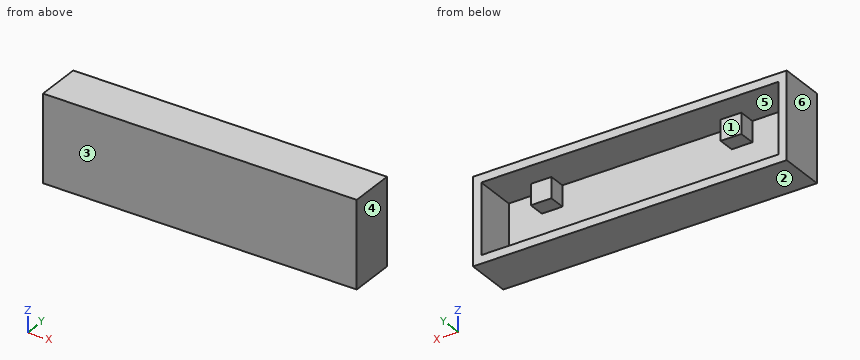
from build123d import *

# Parameters (mm, degrees)
SKETCH1_W           = 76
SKETCH1_H           = 21
SKETCH1_W_2         = 72
SKETCH1_H_2         = 17
BOSS_EXTRUDE1_DEPTH = 10
SKETCH2_W           = 76
SKETCH2_H           = 21
BOSS_EXTRUDE2_DEPTH = 1
SKETCH3_W           = 3.936198622
SKETCH3_H           = 4.059160528
SKETCH3_W_2         = 4.339911302
BOSS_EXTRUDE3_DEPTH = 4
SKETCH4_W           = 5
SKETCH4_H           = 5
BOSS_EXTRUDE4_DEPTH = 4


with BuildPart() as part:
    # Sketch1 → Boss-Extrude1 (new body)
    with BuildSketch(Plane(origin=(0, 0, 0), x_dir=(1, 0, 0), z_dir=(0, 1, 0))):
        with Locations((36, 8.5)):
            Rectangle(SKETCH1_W, SKETCH1_H)
        with Locations((36, 8.5)):
            Rectangle(SKETCH1_W_2, SKETCH1_H_2, mode=Mode.SUBTRACT)
    extrude(amount=BOSS_EXTRUDE1_DEPTH)

    # Sketch2 → Boss-Extrude2 (add)
    with BuildSketch(Plane.XZ):
        with Locations((36, -8.5)):
            Rectangle(SKETCH2_W, SKETCH2_H)
    extrude(amount=BOSS_EXTRUDE2_DEPTH)

    # Sketch3 → Boss-Extrude3 (add)
    with BuildSketch(Plane(origin=(0, 0, 0), x_dir=(1, 0, 0), z_dir=(0, 1, 0))):
        with Locations((18.943139302, 14.970419736)):
            Rectangle(SKETCH3_W, SKETCH3_H)
        with Locations((52.653148019, 14.970419736)):
            Rectangle(SKETCH3_W_2, SKETCH3_H)
    extrude(amount=BOSS_EXTRUDE3_DEPTH)

    # Sketch4 → Boss-Extrude4 (add)
    with BuildSketch(Plane(origin=(0, 0, 0), x_dir=(1, 0, 0), z_dir=(0, 1, 0))):
        with Locations((15.5, 2.5)):
            Rectangle(SKETCH4_W, SKETCH4_H)
        with Locations((61.5, 2.5)):
            Rectangle(SKETCH4_W, SKETCH4_H)
    extrude(amount=BOSS_EXTRUDE4_DEPTH)


solid = part.part
CAD build for the part. Positions are in the model's coordinates, mm. Face numbers are marked on the shaded views. A direction names the side the tool comes from. Give positions to 0.01 mm unless a question says otherwise; leave off trailing zeros. Write each loop counter-clockwise with the first axis right and the second up, starting at its lowest first coordinate (ties: lowest second). Pieces come first, ordered by that corner, then holes. Notation, with made-up numbers: (1.25, 59.5) -> (51.25, 59.5) arc R23 cw to (51.25, 89.5) -> close; hole circle Ø4 at (32, -23.5). An arc over 180 degrees is marked (long way). Return JSON: item names as keys, results as strings.
Item 1: Drop flat-ended pins along their axis: pin 1 (4.5 mm diameter, centred on x = 53.5, z = -15, fed in from +Y); pin 2 (5.5 mm diameter, centred on x = 15, z = -3.5, fed in from +Y); pin 3 (6 mm diameter, centred on x = 38, z = -3.5, fed in from +Y). Give the stop position or say it passes through.
Answer below:
{"pin 1": "stops at y = 10", "pin 2": "stops at y = 4", "pin 3": "stops at y = 0"}
Item 2: Drill centre lines: probe 1 along X at (y, z) = (1.5, -16.25); probe 2 along X at (y, z) = (3.75, -2.75); probe 3 along Z at (x, y) = (51, 3.5). Where is each one in solid material? Low to high.
Answer below:
{"probe 1": "x = -2 to 0, 16.98 to 20.91, 50.48 to 54.82, 72 to 74", "probe 2": "x = -2 to 0, 13 to 18, 59 to 64, 72 to 74", "probe 3": "z = -19 to -12.94, 0 to 2"}
Item 3: Band-saw the part on D-D (y = 3). List the corners of the cut face in (x, z).
Answer below:
{"outline": "(-2, -19) -> (74, -19) -> (74, 2) -> (-2, 2) -> close; hole (0, -17) -> (16.98, -17) -> (16.98, -12.94) -> (20.91, -12.94) -> (20.91, -17) -> (50.48, -17) -> (50.48, -12.94) -> (54.82, -12.94) -> (54.82, -17) -> (72, -17) -> (72, 0) -> (64, 0) -> (64, -5) -> (59, -5) -> (59, 0) -> (18, 0) -> (18, -5) -> (13, -5) -> (13, 0) -> (0, 0) -> close"}
Item 4: Band-saw the part on C-C (z = -10.25). List the corners of the cut face in (x, y).
Answer below:
{"outline": "(-2, -1) -> (74, -1) -> (74, 10) -> (72, 10) -> (72, 0) -> (0, 0) -> (0, 10) -> (-2, 10) -> close"}
Item 5: Two-plate mould, pull along X, no slides. Class the marked faces 3, 4, 5 and 6: +X half, -X half, draft (parallel to the pull), parting line (faces both ways), or undercut.
Answer below:
{"face 3": "draft", "face 4": "+X half", "face 5": "undercut", "face 6": "-X half"}
Item 6: Tool access for the marked faces 1 and 2: list every direction of +Z, -Z, +X, -X, +Y, -Y with a clear straight run to the whole face (end or side of a thin tool).
Answer below:
{"face 1": "+Y", "face 2": "-Z, +X, -X, +Y, -Y"}
Item 7: Band-saw the part on B-B (x = 25.5). List the corners of the cut face in (y, z), then the cut area to 3 significant figures.
Answer below:
{"outline": "(-1, -19) -> (10, -19) -> (10, -17) -> (0, -17) -> (0, 0) -> (10, 0) -> (10, 2) -> (-1, 2) -> close", "area": "61.0 mm2"}
Item 8: Band-saw the part on A-A (y = 6.75). List the corners of the cut face in (x, z), then the cut area to 3 significant figures.
Answer below:
{"outline": "(-2, -19) -> (74, -19) -> (74, 2) -> (-2, 2) -> close; hole (0, -17) -> (72, -17) -> (72, 0) -> (0, 0) -> close", "area": "372 mm2"}
